Geometry check sheet. Reference: drawing and pictorial views, mm from the part's lowest x, y, z. Give positions to 0.01 mm unless a question says otherwise; leave off trailing zeros. Write each loop counter-clockwise with the first axis right and the second up, starting at its lowest first coordinate (ties: lowest second). Pieces come first, ordered by that corner, then holes.
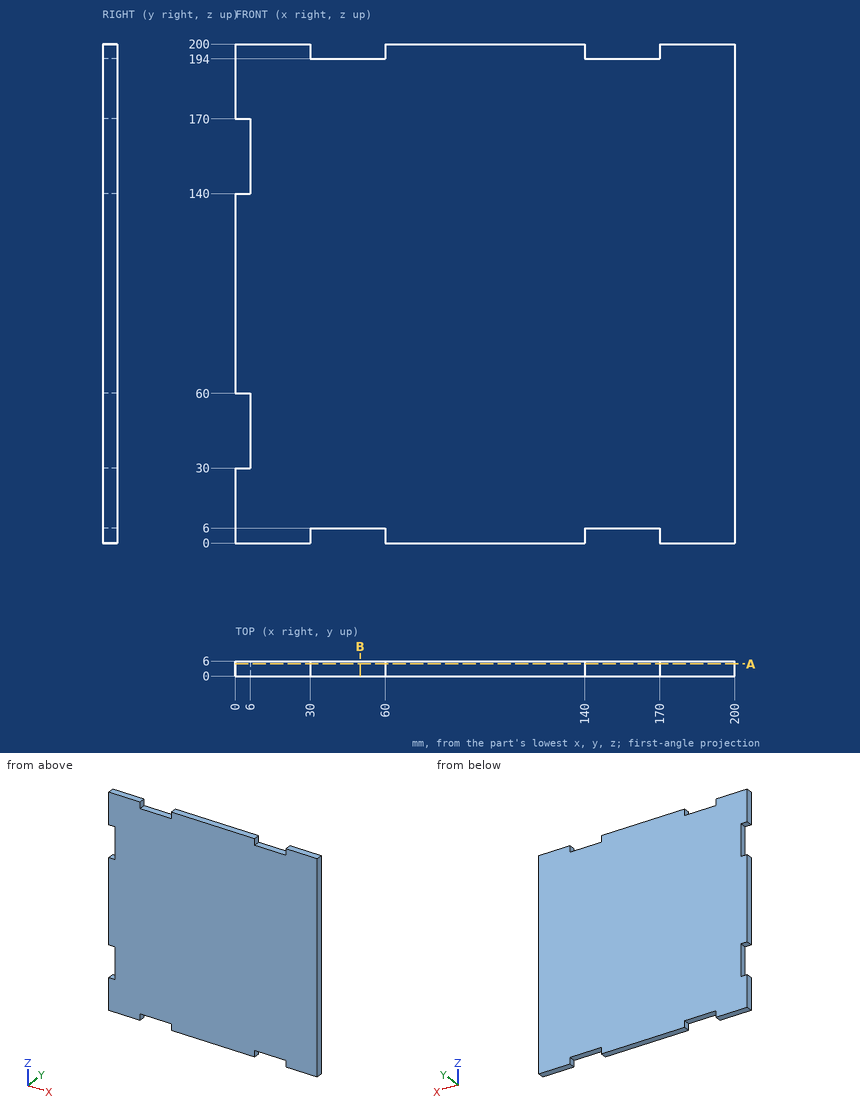
Item 1: Sectioned sample at B-B on x = 50. Record the cut outline in (y, z), then the cut area to 3 significant figures.
Answer key:
outline: (0, 6) - (6, 6) - (6, 194) - (0, 194) - close
area: 1,130 mm2
Item 2: Sectioned sample at A-A on y = 4.9. Record the cut outline in (x, z), then the cut area to 3 significant figures.
Answer key:
outline: (0, 0) - (30, 0) - (30, 6) - (60, 6) - (60, 0) - (140, 0) - (140, 6) - (170, 6) - (170, 0) - (200, 0) - (200, 200) - (170, 200) - (170, 194) - (140, 194) - (140, 200) - (60, 200) - (60, 194) - (30, 194) - (30, 200) - (0, 200) - (0, 170) - (6, 170) - (6, 140) - (0, 140) - (0, 60) - (6, 60) - (6, 30) - (0, 30) - close
area: 38,900 mm2
Item 3: Scan lines: line 1 along Z through (x, y) = (155, 3.1); line 2 along X through (y, z) = (0.65, 33.5). Record each from-to range of solid material in increasing order.
Answer key:
line 1: z = 6 to 194
line 2: x = 6 to 200
Item 4: Depth check by flat-ended pin: pin 1 (1.8 mm diameter, centred on x = 157.5, y = 2, fed in from +Z). Enter the tip coordinate at first touch or a pass-through.
Answer key:
pin 1: stops at z = 194
